from build123d import *

# Parameters (mm, degrees)
DODANIE_WYCI_GNI_CIE1_DEPTH = 6
DODANIE_WYCI_GNI_CIE2_DEPTH = 2
SKORUPA1_T                  = -2
SZKIC3_R                    = 1.7499999999999998
SZKIC3_R_2                  = 1.7500000000000004
SZKIC3_R_3                  = 5
WYTNIJ_WYCI_GNI_CIE1_DEPTH  = 2
ZAOKR_GLENIE1_R             = 3
ZAOKR_GLENIE2_R             = 2
WYTNIJ_WYCI_GNI_CIE2_REACH  = 85.53
SZKIC4_R                    = 1.2500000000000009


with BuildPart() as part:
    # Szkic1 → Dodanie-wyciągnięcie1 (new body)
    with BuildSketch(Plane.XY):
        with BuildLine():
            Line((-37.5, 21.499999999999993), (37.5, 21.499999999999993))
            Line((37.5, 21.499999999999993), (37.5, -21.500000000000004))
            ThreePointArc((37.5, -21.500000000000004), (1.312e-14, -28.797518911304223), (-37.49999999999999, -21.500000000000004))
            Line((-37.49999999999999, -21.500000000000004), (-37.5, 21.499999999999993))
        make_face()
    extrude(amount=DODANIE_WYCI_GNI_CIE1_DEPTH)

    # Szkic2 → Dodanie-wyciągnięcie2 (add)
    with BuildSketch(Plane.XY.offset(6)):
        with BuildLine():
            Line((-40.5, -20.229187385635353), (-40.5, 21.49999999999997))
            ThreePointArc((-40.5, 21.49999999999997), (-39.62132034355964, 23.62132034355963), (-37.49999999999998, 24.49999999999999))
            Line((-37.49999999999998, 24.49999999999999), (37.49999999999998, 24.49999999999999))
            ThreePointArc((37.49999999999998, 24.49999999999999), (39.621320343559645, 23.621320343559635), (40.5, 21.49999999999997))
            Line((40.5, 21.49999999999997), (40.50000000000001, -20.229187385635377))
            ThreePointArc((40.50000000000001, -20.229187385635377), (-9.09e-15, -28.797518911304223), (-40.5, -20.229187385635353))
        make_face()
    extrude(amount=DODANIE_WYCI_GNI_CIE2_DEPTH)

    # Skorupa1
    skorupa1_openings = [part.faces().sort_by_distance(p)[0] for p in [
        (0, -2.499693037, 0),
    ]]
    offset(amount=SKORUPA1_T, openings=skorupa1_openings, kind=Kind.INTERSECTION)

    # Szkic3 → Wytnij-wyciągnięcie1 (cut)
    with BuildSketch(Plane(origin=(0, 0, 6), x_dir=(-1, 0, 0), z_dir=(0, 0, -1))):
        with Locations((-29.5, 13.49999999999999)):
            Circle(SZKIC3_R)
        with Locations((29.5, 13.49999999999999)):
            Circle(SZKIC3_R)
        with Locations((29.5, -14.141648443529768)):
            Circle(SZKIC3_R_2)
        with Locations((-29.5, -14.141648443529768)):
            Circle(SZKIC3_R_2)
        Circle(SZKIC3_R_3)
    extrude(amount=-WYTNIJ_WYCI_GNI_CIE1_DEPTH, mode=Mode.SUBTRACT)

    # Zaokrąglenie1
    zaokr_glenie1_edges = [part.edges().sort_by_distance(p)[0] for p in [
        (-35.5, -20.14164844352976, 3),
        (35.5, -20.14164844352979, 3),
        (35.5, 19.499999999999993, 3),
        (-35.5, 19.499999999999993, 3),
        (-37.499999999999986, -21.5, 3),
        (-37.5, 21.499999999999993, 3),
        (37.5, 21.499999999999993, 3),
        (37.5, -21.499999999999993, 3),
    ]]
    fillet(zaokr_glenie1_edges, radius=ZAOKR_GLENIE1_R)

    # Zaokrąglenie2
    zaokr_glenie2_edges = [part.edges().sort_by_distance(p)[0] for p in [
        (-35.5, -0.7826871340449166, 6),
        (1.421e-14, -26.797518911304223, 6),
        (0, 19.499999999999993, 6),
        (35.5, -0.7826871340449308, 6),
        (-34.621320343559645, 18.621320343559635, 6),
        (34.621320343559645, 18.621320343559635, 6),
        (34.95753406572738, -19.785992272119067, 6),
        (-34.95753406572737, -19.785992272119046, 6),
    ]]
    fillet(zaokr_glenie2_edges, radius=ZAOKR_GLENIE2_R)

    # Wytnij-wyciągnięcie2: up to this face of the body (flat: up to its plane)
    wytnij_wyci_gni_cie2_end = Plane(part.part.faces().sort_by_distance((37.5, -0.477420367, 3))[0])
    # Szkic4 → Wytnij-wyciągnięcie2 (cut, up to the picked face)
    with BuildSketch(Plane.ZY.offset(37.5), mode=Mode.PRIVATE) as wytnij_wyci_gni_cie2_sk1:
        with Locations(Location((2.999999999998171, -5.500000000000033, 0), (0, 0, 323.130102354))):
            Circle(SZKIC4_R)
    wytnij_wyci_gni_cie2_tool1 = split(extrude(wytnij_wyci_gni_cie2_sk1.sketch, amount=-WYTNIJ_WYCI_GNI_CIE2_REACH, mode=Mode.PRIVATE), bisect_by=wytnij_wyci_gni_cie2_end, keep=Keep.BOTH, mode=Mode.PRIVATE)
    add(wytnij_wyci_gni_cie2_tool1.solids().sort_by(Axis((-37.5, -5.5, 3), (1, 1.6e-16, 0)))[0], mode=Mode.SUBTRACT)


solid = part.part
Work out the finished part from the listing and answer in its coordinate system (mm). A direction names the side the tool comes from. Coordinates: 2 decimals unless noted, no trailing zeros. Loops run counter-clockwise (first coordinate to the right, second up) from the corner with the lowest first, then second, coordinate; pieces in that order, holes last. Notation, with made-up numbers: M -15,49 L -8,49 A22 ccw -8,73 Z; hole C -20,29.25 d10. An arc over 180 degrees is marked long. Answer in a Markdown table with one row per item. Add a question column.
1. Flat-ended cylindrical pins translate along their axes: P1, Ø3, axis at y = 0, z = 2.5, coming from the -X side; P2, Ø12.5, axis at x = 6, y = -9, coming from the -Z side; P3, Ø4.5, axis at x = 15.5, z = 2.5, coming from the -Y side; P4, Ø4, axis at x = -14.5, z = 5, coming from the +Y side. Find the tip coordinate at first contact, or state that the pin passes through.
2. A tool of negligible diameter and unlimited length cuts with its end or side. For faces 5 (the cylindrical face through (36.64, 20.6, 3.04)), 6 (the flat face through (35.5, -1, 2)), 7 (the flat face through (0, 21.5, 3)), 8 (the cylindrical face through (36.955, -21.178, 3.042)), from which of +Z, -Z, +X, -X, +Y, -Y can it reach the whole face along a straight path? Write none if from no direction.
3. Consider L1, parallel to X at y = 13.5, z = 7.2; L2, parallel to X at y = 12, z = 2.5; L3, parallel to Y at x = -29.5, z = 6.7. Determine where each line is inside the solid, lowest interval first.
4. Find section C-C, the plane x = -29.5. State how many separate pieces and enclosed holes the cut face has, then the cut area to 3 significant figures.
5. Find section B-B, the plane y = 13.5. Write down the section's boundary in (x, z), then the cut area to 3 significant figures.
6. The mould has two halves that part along Y. Classify faces 1 (the flat face through (-37.5, -1, 3)), 2 (the cylindrical face through (0.45, 18.9, 5.43)), 3 (the cylindrical face through (-36.64, 20.6, 3.04)), 4 (the cylindrical face through (34.9, -1.02, 5.43)): pulls with the +Y half, pulls with the -Y half, needs draft (parallel to the pull), parting line crosses it, or undercut.
7. Find section A-A, the plane z = 3. Write down the section's boundary in (x, y), then the cut area to 3 significant figures.
Reported:
| question | item | result |
|---|---|---|
| 1 | P1 | stops at x = -37.5 |
| 1 | P2 | stops at z = 6 |
| 1 | P3 | stops at y = -27.92 |
| 1 | P4 | stops at y = 24.5 |
| 2 | face 5 | -Z, +X, +Y |
| 2 | face 6 | -Z |
| 2 | face 7 | -Z, +X, -X, +Y |
| 2 | face 8 | -Z, +X, -Y |
| 3 | L1 | x = -40.5 to -31.25, -27.75 to 27.75, 31.25 to 40.5 |
| 3 | L2 | x = -37.5 to -35.5, 35.5 to 37.5 |
| 3 | L3 | y = -24.35 to -15.89, -12.39 to 11.75, 15.25 to 24.5 |
| 4 | separate pieces | 3 |
| 4 | enclosed holes | 0 |
| 4 | area | 110 mm^2 |
| 5 | outline | M -40.5,6 L -37.5,6 L -37.5,0 L -35.5,0 L -35.5,4 A2 cw -33.5,6 L -31.25,6 L -31.25,8 L -40.5,8 Z; M -27.75,6 L 27.75,6 L 27.75,8 L -27.75,8 Z; M 31.25,6 L 33.5,6 A2 cw 35.5,4 L 35.5,0 L 37.5,0 L 37.5,6 L 40.5,6 L 40.5,8 L 31.25,8 Z |
| 5 | area | 174 mm^2 |
| 6 | face 1 | needs draft |
| 6 | face 2 | undercut |
| 6 | face 3 | pulls with the +Y half |
| 6 | face 4 | undercut |
| 7 | outline | M -37.5,-19.45 A3 ccw -35.57,-22.26 A100 ccw 35.57,-22.26 A3 ccw 37.5,-19.45 L 37.5,-6.75 L 35.5,-6.75 L 35.5,-18.07 A3 cw 33.53,-20.88 A98 cw -33.53,-20.88 A3 cw -35.5,-18.07 L -35.5,-6.75 L -37.5,-6.75 Z; M -37.5,-4.25 L -35.5,-4.25 L -35.5,16.5 A3 cw -32.5,19.5 L 32.5,19.5 A3 cw 35.5,16.5 L 35.5,-4.25 L 37.5,-4.25 L 37.5,18.5 A3 ccw 34.5,21.5 L -34.5,21.5 A3 ccw -37.5,18.5 Z |
| 7 | area | 451 mm^2 |
